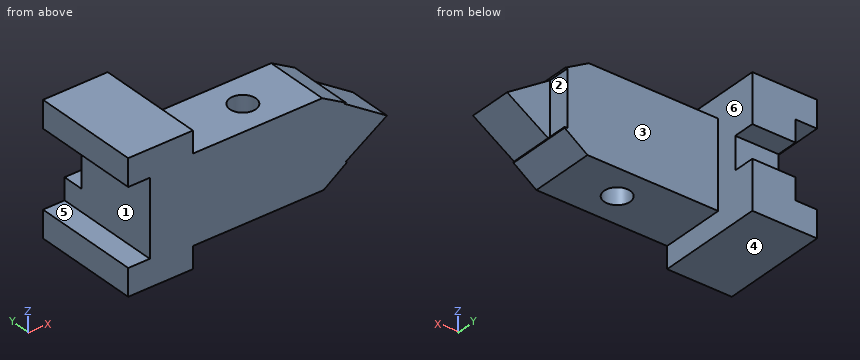
```python
from build123d import *

# Parameters (mm, degrees)
SKETCH1_W           = 30
SKETCH1_H           = 50
BOSS_EXTRUDE1_DEPTH = 60
SKETCH2_W           = 40
SKETCH2_H           = 30
BOSS_EXTRUDE2_DEPTH = 90
SKETCH3_R           = 6
CUT_EXTRUDE1_DEPTH  = 90
CUT_EXTRUDE3_DEPTH  = 90
SKETCH6_W           = 25.687042716
SKETCH6_H           = 10
CUT_EXTRUDE4_DEPTH  = 20
SKETCH7_W           = 18.776678674
SKETCH7_H           = 30
CUT_EXTRUDE5_DEPTH  = 6
SKETCH8_W           = 18.776678674
SKETCH8_H           = 30
CUT_EXTRUDE6_DEPTH  = 1
SKETCH9_W           = 18.776678674
SKETCH9_H           = 30
CUT_EXTRUDE7_DEPTH  = 8
CUT_EXTRUDE8_DEPTH  = 48
SKETCH11_W          = 20
SKETCH11_H          = 15
CUT_EXTRUDE9_DEPTH  = 10
SKETCH12_W          = 10
SKETCH12_H          = 35.03931538
CUT_EXTRUDE10_DEPTH = 70


with BuildPart() as part:
    # Sketch1 → Boss-Extrude1 (new body)
    with BuildSketch(Plane.XY):
        with Locations((-6.834061135, 8.187772926)):
            Rectangle(SKETCH1_W, SKETCH1_H)
    extrude(amount=-BOSS_EXTRUDE1_DEPTH)

    # Sketch2 → Boss-Extrude2 (add)
    with BuildSketch(Plane(origin=(8.165938865, 0, 0), x_dir=(0, 0, -1), z_dir=(1, 0, 0))):
        with Locations((30, -1.812227074)):
            Rectangle(SKETCH2_W, SKETCH2_H)
    extrude(amount=BOSS_EXTRUDE2_DEPTH)

    # Sketch3 → Cut-Extrude1 (cut)
    with BuildSketch(Plane.XY.offset(-10)):
        with Locations((43.165938865, -1.812227074)):
            Circle(SKETCH3_R)
    extrude(amount=-CUT_EXTRUDE1_DEPTH, mode=Mode.SUBTRACT)

    # Sketch4 → Cut-Extrude3 (cut)
    with BuildSketch(Plane(origin=(0, 13.187772926, 0), x_dir=(1, 0, 0), z_dir=(0, 1, 0))):
        Polygon((79.389260191, 50), (68.777599528, 50), (79.389260191, 42.463070185), align=None)
        Polygon((79.389260191, 16.479787589), (68.165938865, 10), (79.389260191, 10), align=None)
    extrude(amount=-CUT_EXTRUDE3_DEPTH, mode=Mode.SUBTRACT)

    # Sketch6 → Cut-Extrude4 (cut)
    with BuildSketch(Plane(origin=(98.165938865, 0, 0), x_dir=(0, 0, -1), z_dir=(1, 0, 0))):
        with Locations((29.167914445, 8.187772926)):
            Rectangle(SKETCH6_W, SKETCH6_H)
    extrude(amount=-CUT_EXTRUDE4_DEPTH, mode=Mode.SUBTRACT)

    # Sketch7 → Cut-Extrude5 (cut)
    with BuildSketch(Plane.XY.offset(-10)):
        with Locations((88.777599528, -1.812227074)):
            Rectangle(SKETCH7_W, SKETCH7_H)
    extrude(amount=-CUT_EXTRUDE5_DEPTH, mode=Mode.SUBTRACT)

    # Sketch8 → Cut-Extrude6 (cut)
    with BuildSketch(Plane.XY.offset(-16)):
        with Locations((88.777599528, -1.812227074)):
            Rectangle(SKETCH8_W, SKETCH8_H)
    extrude(amount=-CUT_EXTRUDE6_DEPTH, mode=Mode.SUBTRACT)

    # Sketch9 → Cut-Extrude7 (cut)
    with BuildSketch(Plane(origin=(0, 0, -50), x_dir=(-1, 0, 0), z_dir=(0, 0, -1))):
        with Locations((-88.777599528, -1.812227074)):
            Rectangle(SKETCH9_W, SKETCH9_H)
    extrude(amount=-CUT_EXTRUDE7_DEPTH, mode=Mode.SUBTRACT)

    # Sketch10 → Cut-Extrude8 (cut)
    with BuildSketch(Plane(origin=(0, 3.187772926, 0), x_dir=(1, 0, 0), z_dir=(0, 1, 0))):
        Polygon((98.165938865, 17), (98.165938865, 29.5), (78.165938865, 16.324393087), (79.179406262, 16.358628366), (79.389260191, 16.479787589), (79.389260191, 17), align=None)
        Polygon((79.389260191, 42.011075028), (78.777599528, 42.011435803), (98.165938865, 29.5), (98.165938865, 42), (79.389260191, 42), align=None)
    extrude(amount=-CUT_EXTRUDE8_DEPTH, mode=Mode.SUBTRACT)

    # Sketch11 → Cut-Extrude9 (cut)
    with BuildSketch(Plane(origin=(0, 33.187772926, 0), x_dir=(1, 0, 0), z_dir=(0, 1, 0))):
        with Locations((-1.834061135, 30)):
            Rectangle(SKETCH11_W, SKETCH11_H)
    extrude(amount=-CUT_EXTRUDE9_DEPTH, mode=Mode.SUBTRACT)

    # Sketch12 → Cut-Extrude10 (cut)
    with BuildSketch(Plane(origin=(0, 33.187772926, 0), x_dir=(1, 0, 0), z_dir=(0, 1, 0))):
        with Locations((-16.834061135, 30)):
            Rectangle(SKETCH12_W, SKETCH12_H)
    extrude(amount=-CUT_EXTRUDE10_DEPTH, mode=Mode.SUBTRACT)


solid = part.part
```
The listing builds one solid part. Answer for the finished solid, in the listing's coordinates (mm). Face numbers are marked on the shaded views. A direction names the side the tool comes from. Coordinates: 2 decimals unless noted, no trailing zeros. Write each loop counter-clockwise with the first axis right and the second up, starting at its lowest first coordinate (ties: lowest second). Pieces come first, ordered by that corner, then holes. Notation, with made-up numbers: M 12.25,27 L 55.25,27 A32 ccw 55.25,60 Z; hole C 60,53 d10. An arc over 180 degrees is marked long. Use a Markdown table: item, result. Add a question column.
1. Which of the six approach directions +Z, -Z, +X, -X, +Y, -Y give full straight-line access (tool end or side, diameter ignored) to the marked faces 1, 2 and 3?
2. Given P1, Ø3, axis at y = 6.5, z = -24, coming from the +X side; P2, Ø5, axis at y = -1, z = -37, coming from the +X side; P3, Ø12, axis at y = -1, z = -31.5, coming from the -X side, each flat-ended and moving along its own axis, determine where each tip first touches the part or whether it passes through.
3. Section D-D (y = -5) is taken. Give the vertices of the cut face in (x, z), plus the area to 3 significant figures.
4. Section B-B (z = -39) is taken. Give the vertices of the cut face in (x, y).
5. For a pull along Z with two mould halves and no side action, classify the marked faces 4, 5 and 6 as +Z half, -Z half, draft (parallel to the pull), parting line (faces both ways), or undercut.
6. Section A-A (y = -13) is taken. Give the vertices of the cut face in (x, z), plus the area to 3 significant figures.
7. Section C-C (x = 2.5) is taken. Give the vertices of the cut face in (y, z).
8. Straight lines are drawn through the part: line 1 along X through (y, z) = (26.5, -56); line 2 along X through (y, z) = (17, -15); line 3 along Z through (x, y) = (21.5, 11.5). For each, find the intervals that lie inside material, in ascending order. Write a range as [from, to].
Data:
| question | item | result |
|---|---|---|
| 1 | face 1 | -X, +Y, -Y |
| 1 | face 2 | +X, +Y |
| 1 | face 3 | +Z, -Z, +X, +Y |
| 2 | P1 | stops at x = 78.17 |
| 2 | P2 | stops at x = 90.42 |
| 2 | P3 | stops at x = -11.83 |
| 3 | outline | M -21.83,-60 L 8.17,-60 L 8.17,-50 L 38.08,-50 L 38.08,-10 L 8.17,-10 L 8.17,0 L -21.83,0 L -21.83,-12.48 L -11.83,-12.48 L -11.83,-47.52 L -21.83,-47.52 Z; M 48.25,-50 L 68.78,-50 L 79.39,-42.46 L 79.39,-42.01 L 78.78,-42.01 L 98.17,-29.5 L 78.17,-16.32 L 79.18,-16.36 L 68.17,-10 L 48.25,-10 Z |
| 3 | area | 4,040 mm2 |
| 4 | outline | M -11.83,-16.81 L 83.44,-16.81 L 83.44,3.19 L 78.17,3.19 L 78.17,13.19 L 8.17,13.19 L 8.17,33.19 L -11.83,33.19 Z; hole C 43.17,-1.81 d12 |
| 5 | face 4 | -Z half |
| 5 | face 5 | undercut |
| 5 | face 6 | draft |
| 6 | outline | M -21.83,-60 L 8.17,-60 L 8.17,-50 L 68.78,-50 L 79.39,-42.46 L 79.39,-42.01 L 78.78,-42.01 L 98.17,-29.5 L 78.17,-16.32 L 79.18,-16.36 L 68.17,-10 L 8.17,-10 L 8.17,0 L -21.83,0 L -21.83,-12.48 L -11.83,-12.48 L -11.83,-47.52 L -21.83,-47.52 Z |
| 6 | area | 4,450 mm2 |
| 7 | outline | M -16.81,-60 L 33.19,-60 L 33.19,-37.5 L 23.19,-37.5 L 23.19,-22.5 L 33.19,-22.5 L 33.19,0 L -16.81,0 Z |
| 8 | line 1 | x = [-21.83, 8.17] |
| 8 | line 2 | x = [-11.83, 8.17] |
| 8 | line 3 | z = [-50, -10] |
